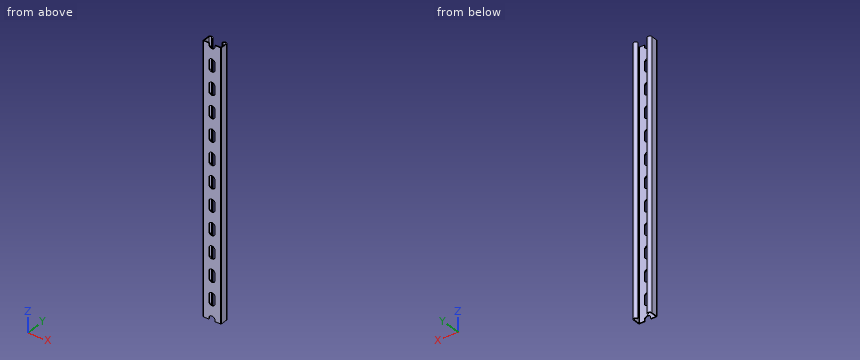
```python
from build123d import *

# Parameters (mm, degrees)
PAD_DEPTH                    = 300
POCKET_DEPTH                 = 3
POCKET_LINEARPATTERN_2_DEPTH = 3
POCKET_LINEARPATTERN_3_DEPTH = 3
POCKET_LINEARPATTERN_4_DEPTH = 3
POCKET_LINEARPATTERN_5_DEPTH = 3
POCKET_LINEARPATTERN_6_DEPTH = 3
POCKET_LINEARPATTERN_7_DEPTH = 3
POCKET_LINEARPATTERN_8_DEPTH = 3


with BuildPart() as part:
    # Sketch → Pad (new body, symmetric)
    with BuildSketch(Plane.XY):
        with BuildLine():
            ThreePointArc((-11.1125, 15.8775), (-15.875, 20.64), (-20.6375, 15.8775))
            Line((-20.6375, 1.5), (-20.6375, 15.8775))
            ThreePointArc((-20.6375, 1.5), (-20.19816, 0.43934), (-19.1375, 0))
            Line((19.1375, 0), (-19.1375, 0))
            ThreePointArc((19.1375, 0), (20.19816, 0.43934), (20.6375, 1.5))
            Line((20.6375, 15.8775), (20.6375, 1.5))
            ThreePointArc((20.6375, 15.8775), (15.875, 20.64), (11.1125, 15.8775))
            Line((11.1125, 15.8775), (13.00988, 15.8775))
            ThreePointArc((18.74012, 15.8775), (15.875, 18.74262), (13.00988, 15.8775))
            Line((18.74012, 15.8775), (18.74012, 2.89738))
            ThreePointArc((17.74012, 1.89738), (18.447227, 2.190273), (18.74012, 2.89738))
            Line((17.74012, 1.89738), (-17.74012, 1.89738))
            ThreePointArc((-18.74012, 2.89738), (-18.447227, 2.190273), (-17.74012, 1.89738))
            Line((-18.74012, 2.89738), (-18.74012, 15.8775))
            ThreePointArc((-13.00988, 15.8775), (-15.875, 18.74262), (-18.74012, 15.8775))
            Line((-13.00988, 15.8775), (-11.1125, 15.8775))
        make_face()
    extrude(amount=PAD_DEPTH, both=True)

    # Sketch001 → Pocket (cut)
    with BuildSketch(Plane.XZ):
        with BuildLine():
            ThreePointArc((7.14375, 7.14125), (0, 14.285), (-7.14375, 7.14125))
            Line((-7.14375, 7.14125), (-7.14375, -7.14125))
            ThreePointArc((-7.14375, -7.14125), (0, -14.285), (7.14375, -7.14125))
            Line((7.14375, -7.14125), (7.14375, 7.14125))
        make_face()
    pocket = extrude(amount=-POCKET_DEPTH, mode=Mode.SUBTRACT)

    # Sketch001 LinearPattern 2 → Pocket LinearPattern 2 (cut)
    with BuildSketch(Plane(origin=(0, 0, 50.8), x_dir=(1, 0, 0), z_dir=(0, -1, 0))):
        with BuildLine():
            ThreePointArc((7.14375, 7.14125), (0, 14.285), (-7.14375, 7.14125))
            Line((-7.14375, 7.14125), (-7.14375, -7.14125))
            ThreePointArc((-7.14375, -7.14125), (0, -14.285), (7.14375, -7.14125))
            Line((7.14375, -7.14125), (7.14375, 7.14125))
        make_face()
    pocket_linearpattern_2 = extrude(amount=-POCKET_LINEARPATTERN_2_DEPTH, mode=Mode.SUBTRACT)

    # Sketch001 LinearPattern 3 → Pocket LinearPattern 3 (cut)
    with BuildSketch(Plane(origin=(0, 0, 101.6), x_dir=(1, 0, 0), z_dir=(0, -1, 0))):
        with BuildLine():
            ThreePointArc((7.14375, 7.14125), (0, 14.285), (-7.14375, 7.14125))
            Line((-7.14375, 7.14125), (-7.14375, -7.14125))
            ThreePointArc((-7.14375, -7.14125), (0, -14.285), (7.14375, -7.14125))
            Line((7.14375, -7.14125), (7.14375, 7.14125))
        make_face()
    pocket_linearpattern_3 = extrude(amount=-POCKET_LINEARPATTERN_3_DEPTH, mode=Mode.SUBTRACT)

    # Sketch001 LinearPattern 4 → Pocket LinearPattern 4 (cut)
    with BuildSketch(Plane(origin=(0, 0, 152.4), x_dir=(1, 0, 0), z_dir=(0, -1, 0))):
        with BuildLine():
            ThreePointArc((7.14375, 7.14125), (0, 14.285), (-7.14375, 7.14125))
            Line((-7.14375, 7.14125), (-7.14375, -7.14125))
            ThreePointArc((-7.14375, -7.14125), (0, -14.285), (7.14375, -7.14125))
            Line((7.14375, -7.14125), (7.14375, 7.14125))
        make_face()
    pocket_linearpattern_4 = extrude(amount=-POCKET_LINEARPATTERN_4_DEPTH, mode=Mode.SUBTRACT)

    # Sketch001 LinearPattern 5 → Pocket LinearPattern 5 (cut)
    with BuildSketch(Plane(origin=(0, 0, 203.2), x_dir=(1, 0, 0), z_dir=(0, -1, 0))):
        with BuildLine():
            ThreePointArc((7.14375, 7.14125), (0, 14.285), (-7.14375, 7.14125))
            Line((-7.14375, 7.14125), (-7.14375, -7.14125))
            ThreePointArc((-7.14375, -7.14125), (0, -14.285), (7.14375, -7.14125))
            Line((7.14375, -7.14125), (7.14375, 7.14125))
        make_face()
    pocket_linearpattern_5 = extrude(amount=-POCKET_LINEARPATTERN_5_DEPTH, mode=Mode.SUBTRACT)

    # Sketch001 LinearPattern 6 → Pocket LinearPattern 6 (cut)
    with BuildSketch(Plane(origin=(0, 0, 254), x_dir=(1, 0, 0), z_dir=(0, -1, 0))):
        with BuildLine():
            ThreePointArc((7.14375, 7.14125), (0, 14.285), (-7.14375, 7.14125))
            Line((-7.14375, 7.14125), (-7.14375, -7.14125))
            ThreePointArc((-7.14375, -7.14125), (0, -14.285), (7.14375, -7.14125))
            Line((7.14375, -7.14125), (7.14375, 7.14125))
        make_face()
    pocket_linearpattern_6 = extrude(amount=-POCKET_LINEARPATTERN_6_DEPTH, mode=Mode.SUBTRACT)

    # Sketch001 LinearPattern 7 → Pocket LinearPattern 7 (cut)
    with BuildSketch(Plane(origin=(0, 0, 304.8), x_dir=(1, 0, 0), z_dir=(0, -1, 0))):
        with BuildLine():
            ThreePointArc((7.14375, 7.14125), (0, 14.285), (-7.14375, 7.14125))
            Line((-7.14375, 7.14125), (-7.14375, -7.14125))
            ThreePointArc((-7.14375, -7.14125), (0, -14.285), (7.14375, -7.14125))
            Line((7.14375, -7.14125), (7.14375, 7.14125))
        make_face()
    pocket_linearpattern_7 = extrude(amount=-POCKET_LINEARPATTERN_7_DEPTH, mode=Mode.SUBTRACT)

    # Sketch001 LinearPattern 8 → Pocket LinearPattern 8 (cut)
    with BuildSketch(Plane(origin=(0, 0, 355.6), x_dir=(1, 0, 0), z_dir=(0, -1, 0))):
        with BuildLine():
            ThreePointArc((7.14375, 7.14125), (0, 14.285), (-7.14375, 7.14125))
            Line((-7.14375, 7.14125), (-7.14375, -7.14125))
            ThreePointArc((-7.14375, -7.14125), (0, -14.285), (7.14375, -7.14125))
            Line((7.14375, -7.14125), (7.14375, 7.14125))
        make_face()
    pocket_linearpattern_8 = extrude(amount=-POCKET_LINEARPATTERN_8_DEPTH, mode=Mode.SUBTRACT)

    # Mirrored: Pocket, Pocket LinearPattern 2, Pocket LinearPattern 3, Pocket LinearPattern 4, Pocket LinearPattern 5, Pocket LinearPattern 6, Pocket LinearPattern 7, Pocket LinearPattern 8 across Sketch001 H_Axis
    add(pocket.mirror(Plane(origin=(0, 0, 0), x_dir=(0, -1, 0), z_dir=(0, 0, 1))), mode=Mode.SUBTRACT)
    add(pocket_linearpattern_2.mirror(Plane(origin=(0, 0, 0), x_dir=(0, -1, 0), z_dir=(0, 0, 1))), mode=Mode.SUBTRACT)
    add(pocket_linearpattern_3.mirror(Plane(origin=(0, 0, 0), x_dir=(0, -1, 0), z_dir=(0, 0, 1))), mode=Mode.SUBTRACT)
    add(pocket_linearpattern_4.mirror(Plane(origin=(0, 0, 0), x_dir=(0, -1, 0), z_dir=(0, 0, 1))), mode=Mode.SUBTRACT)
    add(pocket_linearpattern_5.mirror(Plane(origin=(0, 0, 0), x_dir=(0, -1, 0), z_dir=(0, 0, 1))), mode=Mode.SUBTRACT)
    add(pocket_linearpattern_6.mirror(Plane(origin=(0, 0, 0), x_dir=(0, -1, 0), z_dir=(0, 0, 1))), mode=Mode.SUBTRACT)
    add(pocket_linearpattern_7.mirror(Plane(origin=(0, 0, 0), x_dir=(0, -1, 0), z_dir=(0, 0, 1))), mode=Mode.SUBTRACT)
    add(pocket_linearpattern_8.mirror(Plane(origin=(0, 0, 0), x_dir=(0, -1, 0), z_dir=(0, 0, 1))), mode=Mode.SUBTRACT)


solid = part.part
```
Can you work these out from the model? Positions are in its coordinate system, mm. Coordinates: 2 decimals unless noted, no trailing zeros. Write each loop counter-clockwise with the first axis right and the second up, starting at its lowest first coordinate (ties: lowest second). Pieces come first, ordered by that corner, then holes. Notation, with made-up numbers: (68.5, -37.5) - (126.5, -37.5) arc R3 ccw to (126.5, -33.5) - close; hole circle Ø5 at (53.5, 33.25). An arc over 180 degrees is marked (long way). Return JSON: item names as keys, results as strings.
Q1. Please list where these lines run through material, in increasing order: L1, parallel to Y at x = 16.5, z = -191.5; L2, parallel to X at y = 11.25, z = -202; L3, parallel to X at y = 16.5, z = -33. Write a range as from..to.
Computed values:
{"L1": "y = 0..1.9, 18.67..20.6", "L2": "x = -20.64..-18.74, 18.74..20.64", "L3": "x = -20.6..-18.67, -13.08..-11.15, 11.15..13.08, 18.67..20.6"}
Q2. If we section it at B-B (x = 0): Count the separate pieces of the cut face and the enclosed holes in it, then the cut area to 3 significant figures.
Computed values:
{"separate pieces": "12", "enclosed holes": "0", "area": "506 mm2"}
Q3. I'm going to push flat-ended pins straight in: pin 1 Ø0.6 at (y, z) = (1, 149.5) entering from -X; pin 2 Ø0.6 at (y, z) = (0.5, -298.5) entering from +X; pin 3 Ø1.5 at (x, z) = (-8.5, 205.5) entering from +Y. Where does each tip first touch, or does it pass through?
Computed values:
{"pin 1": "stops at x = -20.62", "pin 2": "stops at x = 20.46", "pin 3": "stops at y = 1.9"}
Q4. If we section it at A-A (y = 7.25): Please give me the cut outline in (x, z).
Computed values:
{"outline": "(-20.64, -300) - (-18.74, -300) - (-18.74, 300) - (-20.64, 300) - close; (18.74, -300) - (20.64, -300) - (20.64, 300) - (18.74, 300) - close"}
